Source: CAD feature listing. Evaluate the final solid. Frame: model axes, mm. Round coordinates to 2 decimals unless told otherwise and drop trailing zeros. Order: outer loops, then holes, each group sorted by start corner. A loop starts at its lowest first (then second) coordinate and runs counter-clockwise, first axis right, second up. Notation, with made-up numbers: (13.5, -34) - (41.5, -34) arc R26 ccw to (41.5, -9) - close; hole circle Ø8 at (69.25, 38.5). An arc over 180 degrees is marked (long way). Return JSON: item names as keys, results as strings. Group by question number.
1) Ray query, line 1 (Z direction, x = 0, y = 1); line 2 (Y direction, x = 61.75, z = 0); line 3 (Z direction, x = 62, y = 72). Return the intervals inside material, ascending. Write a range as from..to.
2) Section A-A, the plane x = -45.5. Return loops of the section in (y, z).
3) Contact query for flat-ended pins moving along their axis: P1, Ø2.5, axis at x = -22.75, z = 39.4, coming from the +Y side; P2, Ø1, axis at x = 0, z = -21.5, coming from the +Y side; P3, Ø1.5, axis at x = 47, z = 6.5, coming from the +Y side; P4, Ø2, axis at y = 14, z = 1.5, coming from the +X side. Output: stop coordinate, or through.
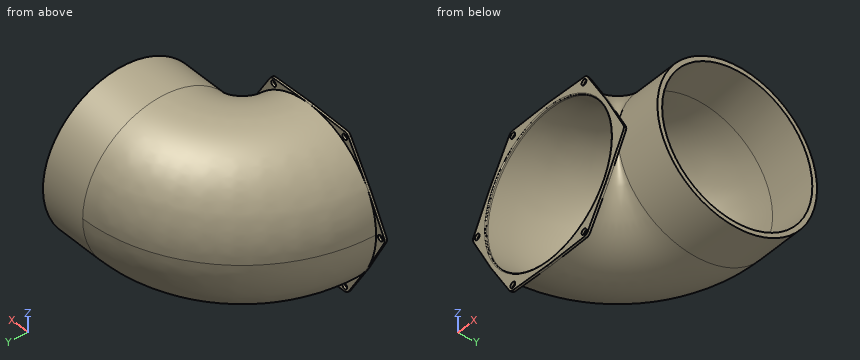
Autodesk Inventor part; units mm, degrees
ref_plane "YZ Plane" through (0, 0, 0) normal (1, 0, 0) x (0, 1, 0)
ref_plane "XZ Plane" through (0, 0, 0) normal (0, 1, 0) x (-1, 0, 0)
ref_plane "XY Plane" through (0, 0, 0) normal (0, 0, 1) x (1, 0, 0)
sketch "Sketch1" plane through (0, 0, 0) normal (0, 1, 0) x (-1, 0, 0)
  circle A0 centre (0, 0) radius 42
  circle A1 centre (0, 0) radius 45.5
  circle A2 centre (45.5, 0) radius 1.524
  circle A3 centre (0, 0) radius 40.7442
  circle A4 centre (0, 0) radius 42.762
  line L0 (40.7442, 0) -> (42.762, 0)
  circle A5 centre (45.5, 0) radius 2.738
  line L1 (47.9085, 1.3023) -> (37.6155, 20.3387)
  line L2 (47.9085, -1.3023) -> (37.6155, -20.3387)
  line L3 (25.082, 40.8388) -> (36.4216, 22.4067)
  circle A6 centre (22.75, 39.4042) radius 2.738
  circle A7 centre (22.75, 39.4042) radius 1.524
  line L4 (22.8264, 42.1411) -> (1.194, 42.7453)
  line L5 (-22.8264, 42.1411) -> (-1.194, 42.7453)
  circle A8 centre (-22.75, 39.4042) radius 2.738
  circle A9 centre (-22.75, 39.4042) radius 1.524
  line L6 (-25.082, 40.8388) -> (-36.4216, 22.4067)
  line L7 (-47.9085, 1.3023) -> (-37.6155, 20.3387)
  circle A10 centre (-45.5, 0) radius 2.738
  circle A11 centre (-45.5, 0) radius 1.524
  line L8 (-47.9085, -1.3023) -> (-37.6155, -20.3387)
  line L9 (-25.082, -40.8388) -> (-36.4216, -22.4067)
  circle A12 centre (-22.75, -39.4042) radius 2.738
  circle A13 centre (-22.75, -39.4042) radius 1.524
  line L10 (-22.8264, -42.1411) -> (-1.194, -42.7453)
  line L11 (22.8264, -42.1411) -> (1.194, -42.7453)
  circle A14 centre (22.75, -39.4042) radius 2.738
  circle A15 centre (22.75, -39.4042) radius 1.524
  line L12 (25.082, -40.8388) -> (36.4216, -22.4067)
  point P0 (21.381, 37.033)
  point P1 (-21.381, 37.033)
  point P2 (-42.762, 0)
  point P3 (-21.381, -37.033)
  point P4 (21.381, -37.033)
  point P5 (-1.194, 42.7453)
  point P6 (-1.194, -42.7453)
  point P7 (1.194, -42.7453)
  dimension "d1" = 91
  dimension "d0" = 84
  dimension "d2" = 3.048
  dimension "d3" = 0.762
  dimension "d6" = 360
extrude "Extrusion1" add sketch "Sketch1" along normal blind 1.27 contours A0 | A2 A1 A5 | A1 A5 A2 | A5 A4 L1 A1 | A1 L1 A5 | A5 L2 A1 | A1 L2 A4 A5 | A4 | L3 A4 A6 A1 | A1 A6 L3 | L12 A14 A1 | A1 A14 A4 L12 | A6 A1 A7 | A1 A7 A6 | A14 A1 A15 | A1 A15 A14 | A4 L4 A1 A6 | A6 A1 L4 | A14 A1 L11 A4 | L11 A1 A14 | A4 A8 A1 L5 | A1 A8 L5 | L10 A1 A12 A4 | L10 A12 A1 | A4 L6 A1 A8 | A8 A1 A9 | A1 A9 A8 | A12 A1 L9 A4 | A12 A1 A13 | A12 A1 A13 | A1 L6 A8 | A12 L9 A1 | A4 A10 A1 L7 | L8 A1 A10 A4 | A10 A1 A11 | A1 A10 L7 | L8 A10 A1 | A1 A11 A10
sketch "Sketch2" plane through (0, 1.27, 0) normal (0, 1, 0) x (1, 0, 0)
  circle A0 centre (0, 0) radius 40.7442
  circle A1 centre (-45.5, 0) radius 1.524
  circle A2 centre (-45.5, 0) radius 2.738
  circle A3 centre (0, 0) radius 42.762
  circle A4 centre (0, 0) radius 40.2362
  line L0 (42.762, -52.0415) -> (42.762, 67.6033)
  dimension "d10" = 0.508
revolve "Revolution1" add sketch "Sketch2" angle 90 about axis through (42.762, 1.27, 52.0415) along (0, 0, -1) contours A0 | A3
sketch "Sketch3" plane through (42.762, 44.032, 0) normal (1, 0, 0) x (0, 0, -1)
  circle A0 centre (0, 0) radius 42.762
  line L0 (-42.762, -42.762) -> (-42.762, 0)
  circle A1 centre (0, 0) radius 40.2362
  line L1 (-40.2362, -42.762) -> (-40.2362, 0)
  point P0 (0, -44.032)
extrude "Extrusion2" add sketch "Sketch3" along normal blind 25.4
sketch "Sketch4" plane through (0, 0, 0) normal (0, -1, 0) x (1, 0, 0)
  arc A0 (43.976, 0) -> (47.024, 0) centre (45.5, 0) ccw
  circle A1 centre (45.5, 0) radius 1.524
  point P0 (0, 0)
  point P1 (43.976, 0)
extrude "Extrusion3" add sketch "Sketch4" against normal up to surface (1.27 mm away)
sketch "Sketch5" plane through (0, 0, 0) normal (0, -1, 0) x (1, 0, 0)
  circle A0 centre (0, 0) radius 40.2362
  circle A1 centre (0, 0) radius 40.7442
extrude "Extrusion4" add sketch "Sketch5" against normal up to surface (1.27 mm away)
fillet "Fillet1" radius 0.508 1 edges at (-40.2362, 0, 0)
properties part number "Dispenser Tip_3DPrint"
Geometry check:
{
 "1": {"line 1": "-42.76..-40.24, 40.24..42.76", "line 2": "1.27..3.8, 84.27..86.79", "line 3": "-32.35..-28.93, 28.93..32.35"},
 "2": {"outline": "(0, -5.76) - (1.27, -5.76) - (1.27, -1.52) - (0, -1.52) - close; (0, 1.52) - (1.27, 1.52) - (1.27, 5.76) - (0, 5.76) - close"},
 "3": {"P1": "through", "P2": "y = 69.02", "P3": "y = 86.41", "P4": "x = -39.06"}
}
